Autodesk Inventor part; units mm, degrees
ref_plane "XZ Plane" through (0, 0, 0) normal (0, 1, 0) x (-1, 0, 0)
ref_plane "XY Plane" through (0, 0, 0) normal (0, 0, 1) x (1, 0, 0)
sketch "Sketch3" plane through (0, 0, 0) normal (1, 0, 0) x (0, 1, 0)
  line L0 (0, -2.6) -> (0, 15.6)
  line L1 (-33.9, 0) -> (203.4, 0)
  line L2 (0, 13) -> (169.5, 13)
  line L3 (169.5, 13) -> (169.5, 10)
  line L4 (169.5, 10) -> (25, 10)
  line L5 (25, 10) -> (25, 0)
  line L6 (0, 13) -> (0, 0)
  line L7 (25, 0) -> (0, 0)
  point P0 (0, 13)
  dimension "d10" = 169.5
  dimension "d13" = 10
  dimension "d14" = 13
  dimension "d15" = 25
  dimension "d17" = 3
revolve "Revolution1" add sketch "Sketch3" angle 360 about axis through (0, -10, 0) along (0, 1, 0)
ref_plane "Work Plane1" through (-13, 84.75, 0) normal (1, 0, 0) x (0, 1, 0)
sketch "Sketch4" plane through (-13, 84.75, 0) normal (1, 0, 0) x (0, 1, 0)
  line L0 (-84.75, -13) -> (-84.75, 13)
  line L1 (-118.65, 0) -> (118.65, 0)
  point P0 (-84.75, 0)
  point P1 (-74.75, 0)
  dimension "d18" = 10
hole "Hole1" at (-13, 10, 0) direction (1, 0, 0) diameter 6 end through all
sketch "Sketch5" plane through (0, 169.5, 0) normal (0, 1, 0) x (1, 0, 0)
  circle A0 centre (0, 0) radius 10
  circle A1 centre (0, -10) radius 2.25
  line L0 (0, 18.2) -> (0, -18.2)
  point P0 (2.2357, -9.7469)
  point P1 (-2.2357, -9.7469)
  dimension "d26" = 4.5
extrude "Extrusion3" cut sketch "Sketch5" against normal up to surface (144.5 mm away) contours A1 L0 A0 | A0 L0 A1 picked at (0.5757, -10.6663) picked at (-0.5973, -10.6555)
pattern_circular "Circular Pattern1" count 4 over 360 about axis through (0, 97.25, 0) along (0, 1, 0) of "Extrusion3"
properties part number "Soporte de Marcador"
Input: part model. Units: mm. Frame: model coordinates. A direction names the side the tool comes from. Coordinates: 2 decimals unless noted, no trailing zeros. Write each loop counter-clockwise with the first axis right and the second up, starting at its lowest first coordinate (ties: lowest second). Pieces come first, ordered by that corner, then holes.
1) Pin query (flat end, axial travel): pin 1 Ø6 at (y, z) = (101.5, -9.5) entering from -X; pin 2 Ø3 at (x, z) = (-5, -5) entering from +Y; pin 3 Ø5 at (x, y) = (-8.5, 148) entering from +Z. Return the tip coordinate at first contact, or that it passes through.
2) Section A-A on y = 136. Output: boundary loops of the cut face in (x, z), and give its area (3 significant figures).
3) Section D-D on y = 10. Output: boundary loops of the cut face in (x, z).
4) Material intervals for line 1 along Y through (x, z) = (-6.25, 0); line 2 along X through (y, z) = (55.5, -4); line 3 along X through (y, z) = (77.5, 10.75), sorted ascending.
5) Section C-C on z = 0. Output: boundary loops of the cut face in (x, y), and give its area (3 significant figures).
6) Mould query, pull axis Z, two halves, no side actions, for faces 1 (the cylindrical face through (12.25, 98.26, 0.05)), 2 (the flat face through (0, 0, 0)), 3 (the cylindrical face through (3.9, 85.9, 12.4)). Classes: pulls with the +Z half, pulls with the -Z half, needs draft (parallel to the pull), parting line crosses it, or undercut.
7) Set-up query: faces 4 (the flat face through (-10, 169.5, -3)), 5 (the cylindrical face through (7.015, 96.238, -7.126)). Return all of +Z, -Z, +X, -X, +Y, -Y with unobstructed straight access to the full face (end or side cutting, diameter ignored); none if empty.
8) Section B-B on x = 0. Output: boundary loops of the cut face in (y, z), and give its area (3 significant figures).
Check result:
1. pin 1: stops at x = -11.26
1. pin 2: stops at y = 25
1. pin 3: stops at z = 11.53
2. outline: circle Ø26 at (0, 0); hole (-9.75, -2.24) arc R10 ccw to (-2.24, -9.75) arc R2.25 ccw (long way) to (2.24, -9.75) arc R10 ccw to (9.75, -2.24) arc R2.25 ccw (long way) to (9.75, 2.24) arc R10 ccw to (2.24, 9.75) arc R2.25 ccw (long way) to (-2.24, 9.75) arc R10 ccw to (-9.75, 2.24) arc R2.25 ccw (long way) to start
2. area: 183 mm2
3. outline: (-12.65, -3) arc R13 ccw to (12.65, -3) - close; (-12.65, 3) - (12.65, 3) arc R13 ccw to start
4. line 1: y = 0 to 7, 13 to 25
4. line 2: x = -12.37 to -9.17, 9.17 to 12.37
4. line 3: x = -7.31 to -2.12, 2.12 to 7.31
5. outline: (-13, 0) - (13, 0) - (13, 7) - (-13, 7) - close; (-13, 13) - (13, 13) - (13, 169.5) - (12.25, 169.5) - (12.25, 25) - (-12.25, 25) - (-12.25, 169.5) - (-13, 169.5) - close
5. area: 711 mm2
6. face 1: undercut
6. face 2: needs draft
6. face 3: parting line crosses it
7. face 4: +Z, -Z, +X, -X, +Y
7. face 5: +Y
8. outline: (0, -13) - (169.5, -13) - (169.5, -12.25) - (25, -12.25) - (25, 12.25) - (169.5, 12.25) - (169.5, 13) - (0, 13) - close; hole circle Ø6 at (10, 0)
8. area: 838 mm2
